Geometry check sheet. Reference: the model listing, model coordinates, mm. A direction names the side the tool comes from. Round coordinates to 2 decimals unless told otherwise and drop trailing zeros. Order: outer loops, then holes, each group sorted by start corner. A loop starts at its lowest first (then second) coordinate and runs counter-clockwise, first axis right, second up.
```python
from build123d import *

# Parameters (mm, degrees)
CYLINDER003_R     = 3
CYLINDER003_DEPTH = 148
BOX013_W          = 16
BOX013_H          = 6
BOX013_DEPTH      = 10
CYLINDER002_R     = 3
CYLINDER002_DEPTH = 148
BOX012_W          = 16
BOX012_H          = 6
BOX012_DEPTH      = 10
BOX011_W          = 12
BOX011_H          = 10
BOX011_DEPTH      = 20
BOX010_W          = 25
BOX010_H          = 25
BOX010_DEPTH      = 15
BOX009_W          = 145
BOX009_H          = 170
BOX009_DEPTH      = 200
BOX008_W          = 155
BOX008_H          = 180
BOX008_DEPTH      = 170


with BuildPart() as cylinder003:
    # Cylinder003 → Cylinder003 (new body)
    with BuildSketch(Plane(origin=(7, 139, 175), x_dir=(1, 0, 0), z_dir=(0, -1, 0))):
        Circle(CYLINDER003_R)
    extrude(amount=CYLINDER003_DEPTH)


with BuildPart() as obj1:
    # Box013 → Box013 (new body)
    with BuildSketch(Plane.XY.offset(170)):
        with Locations((8, 3)):
            Rectangle(BOX013_W, BOX013_H)
    extrude(amount=BOX013_DEPTH)

    # Cut010: cut Cylinder003
    add(cylinder003.part, mode=Mode.SUBTRACT)


with BuildPart() as cylinder002:
    # Cylinder002 → Cylinder002 (new body)
    with BuildSketch(Plane(origin=(7, 192, 175), x_dir=(1, 0, 0), z_dir=(0, -1, 0))):
        Circle(CYLINDER002_R)
    extrude(amount=CYLINDER002_DEPTH)


with BuildPart() as obj2:
    # Box012 → Box012 (new body)
    with BuildSketch(Plane(origin=(0, 174, 170), x_dir=(1, 0, 0), z_dir=(0, 0, 1))):
        with Locations((8, 3)):
            Rectangle(BOX012_W, BOX012_H)
    extrude(amount=BOX012_DEPTH)

    # Cut009: cut Cylinder002
    add(cylinder002.part, mode=Mode.SUBTRACT)


with BuildPart() as cube006:
    # Box011 → Box011 (new body)
    with BuildSketch(Plane(origin=(146, 85, 130), x_dir=(1, 0, 0), z_dir=(0, 0, 1))):
        with Locations((6, 5)):
            Rectangle(BOX011_W, BOX011_H)
    extrude(amount=BOX011_DEPTH)


with BuildPart() as agujero001:
    # Box010 → Box010 (new body)
    with BuildSketch(Plane(origin=(10, -7, 5), x_dir=(1, 0, 0), z_dir=(0, 0, 1))):
        with Locations((12.5, 12.5)):
            Rectangle(BOX010_W, BOX010_H)
    extrude(amount=BOX010_DEPTH)


with BuildPart() as cube005:
    # Box009 → Box009 (new body)
    with BuildSketch(Plane(origin=(5, 5, 5), x_dir=(1, 0, 0), z_dir=(0, 0, 1))):
        with Locations((72.5, 85)):
            Rectangle(BOX009_W, BOX009_H)
    extrude(amount=BOX009_DEPTH)


with BuildPart() as caja002:
    # Box008 → Box008 (new body)
    with BuildSketch(Plane.XY):
        with Locations((77.5, 90)):
            Rectangle(BOX008_W, BOX008_H)
    extrude(amount=BOX008_DEPTH)

    # Cut006: cut Cube005
    add(cube005.part, mode=Mode.SUBTRACT)

    # Cut007: cut Agujero001
    add(agujero001.part, mode=Mode.SUBTRACT)

    # Cut008: cut Cube006
    add(cube006.part, mode=Mode.SUBTRACT)

    # Fusion003: union obj2
    add(obj2.part)

    # Fusion004: union obj1
    add(obj1.part)


solid = caja002.part
```
(1) Depth check by flat-ended pin: P1, Ø1.5, axis at x = 2.5, y = 123.5, coming from the +Z side; P2, Ø3, axis at y = 3.5, z = 177, coming from the +X side. Enter the tip coordinate at first touch or a pass-through.
Returned:
P1: stops at z = 170
P2: stops at x = 16
(2) Draft check along X on faces 4 (the flat face through (22, 3, 20)), 5 (the flat face through (152, 95, 140)), 6 (the flat face through (0, 89, 89)). Enter one of: released by +X, released by -X, zero draft, split by the parting line, or undercut.
Returned:
face 4: undercut
face 5: zero draft
face 6: released by -X
(3) Sectioned sample at B-B, the plane z = 175. Record the cut outline in (x, y).
Returned:
outline: (0, 0) - (4, 0) - (4, 6) - (0, 6) - close; (0, 174) - (4, 174) - (4, 180) - (0, 180) - close; (10, 0) - (16, 0) - (16, 6) - (10, 6) - close; (10, 174) - (16, 174) - (16, 180) - (10, 180) - close
(4) Sectioned sample at A-A, the plane z = 112.5. Record the cut outline in (x, y), and give its area (3 significant figures).
Returned:
outline: (0, 0) - (155, 0) - (155, 180) - (0, 180) - close; hole (5, 5) - (150, 5) - (150, 175) - (5, 175) - close
area: 3,250 mm2
(5) Material ranges on line 1 (X direction, y = 99.5, z = 34.5); line 2 (Y direction, x = 34.5, z = 77); line 3 (X direction, y = 176, z = 175), recorded low to high.
Returned:
line 1: x = 0 to 5, 150 to 155
line 2: y = 0 to 5, 175 to 180
line 3: x = 0 to 4, 10 to 16
(6) Sectioned sample at C-C, the plane y = 158.5. Record the cut outline in (x, z), and give its area (4 significant figures).
Returned:
outline: (0, 0) - (155, 0) - (155, 170) - (150, 170) - (150, 5) - (5, 5) - (5, 170) - (0, 170) - close
area: 2,425 mm2
(7) Set-up check for faces 1 (the flat face through (152, 90, 170)), 2 (the flat face through (2, 91, 170)), 3 (the flat face through (152, 90, 130)): record each of +Z, -Z, +X, -X, +Y, -Y from which the full face is reachable in a straight line by a thin tool's end or side.
Returned:
face 1: +Z, +X, +Y, -Y
face 2: +Z, +X, -X
face 3: +X
(8) Sectioned sample at D-D, the plane x = 97. Record the cut outline in (y, z), and give its area (3 significant figures).
Returned:
outline: (0, 0) - (180, 0) - (180, 170) - (175, 170) - (175, 5) - (5, 5) - (5, 170) - (0, 170) - close
area: 2,550 mm2
